Part model, mm, in its own coordinate system. A direction names the side the tool comes from. Round coordinates to 2 decimals unless told otherwise and drop trailing zeros. Loops run counter-clockwise (first coordinate to the right, second up) from the corner with the lowest first, then second, coordinate; pieces in that order, holes last. Notation, with made-up numbers: (48.5, 15) -> (94.5, 15) arc R25 cw to (94.5, 27) -> close; hole circle Ø8 at (58, -28.75). An arc over 180 degrees is marked (long way). Use a Markdown table: item, result. Add a question column.
Item 1: Probe line 1 (Y direction, x = 104.5, z = 25); line 2 (Y direction, x = 107.5, z = 35); line 3 (X direction, y = 83.5, z = 4.5). List the from-to ranges inside material, lowest first. Write a range as [from, to].
Item 2: Cut at C-C, the plane z = 13. List the corners of the cut face in (x, y), plus the area to 3 significant figures.
Item 3: Flat gauge pins, fed straight in: pin 1 (6.5 mm diameter, centred on y = 85, z = 25, fed in from +X); pin 2 (10.5 mm diameter, centred on y = 85, z = -25, fed in from -X); pin 3 (1.5 mm diameter, centred on x = 6, z = 24, fed in from +Y). Where does each tip first touch, or does it go through?
Item 4: Cut at A-A, the plane y = 95. List the corners of the cut face in (x, z).
Item 5: Cut at D-D, the plane y = 40. List the corners of the cut face in (x, z).
Item 6: Two-plate mould, pull along Z, no slides. Class faces 1 (the face through (28, 9, -40)), 2 (the face through (104.93, 32.11, -33.66)), 3 (the face through (4, 0, 1)), 4 (the face through (28, 9, 40)): pulls with the +Z half, pulls with the -Z half, needs draft (parallel to the pull), parting line crosses it, or undercut.
Item 7: Cut at B-B, the plane z = 35. List the corners of the cut face in (x, y), plus the area to 3 significant figures.
Item 8: Which spindle directions (+Z, -Z, +X, -X, +Y, -Y) get a long thin tool onto all of the face, cutting with end or side? Do faces 5 (the face through (104.93, 97.48, 34.67)), 6 (the face through (-1, 10, -1)). Say none if no direction does.
```python
from build123d import *

# Parameters (mm, degrees)
SKETCH2_W           = 200
SKETCH2_H           = 80
BOSS_EXTRUDE1_DEPTH = 10
SKETCH3_W           = 80
SKETCH3_H           = 100
BOSS_EXTRUDE2_DEPTH = 10
SKETCH6_R           = 4
CUT_EXTRUDE2_DEPTH  = 10
SKETCH8_R           = 2.5
CUT_EXTRUDE3_DEPTH  = 100


with BuildPart() as part:
    # Sketch2 → Boss-Extrude1 (new body)
    with BuildSketch(Plane(origin=(0, 0, 0), x_dir=(1, 0, 0), z_dir=(0, 1, 0))):
        Rectangle(SKETCH2_W, SKETCH2_H)
    extrude(amount=BOSS_EXTRUDE1_DEPTH)

    # Sketch3 → Boss-Extrude2 (add)
    with BuildSketch(Plane(origin=(100, 0, 0), x_dir=(0, 0, -1), z_dir=(1, 0, 0))):
        with Locations((0, 50)):
            Rectangle(SKETCH3_W, SKETCH3_H)
    extrude(amount=BOSS_EXTRUDE2_DEPTH)

    # Sketch6 → Cut-Extrude2 (cut)
    with BuildSketch(Plane.ZY.offset(-100)):
        with Locations((-25, 85)):
            Circle(SKETCH6_R)
        with Locations((25, 85)):
            Circle(SKETCH6_R)
        with Locations((-25, 40)):
            Circle(SKETCH6_R)
        with Locations((25, 40)):
            Circle(SKETCH6_R)
    extrude(amount=-CUT_EXTRUDE2_DEPTH, mode=Mode.SUBTRACT)

    # Sketch8 → Cut-Extrude3 (cut)
    with BuildSketch(Plane.ZY.offset(-100)):
        with Locations((-35, 95)):
            Circle(SKETCH8_R)
        with Locations((35, 95)):
            Circle(SKETCH8_R)
        with Locations((-35, 30)):
            Circle(SKETCH8_R)
        with Locations((35, 30)):
            Circle(SKETCH8_R)
    extrude(amount=-CUT_EXTRUDE3_DEPTH, mode=Mode.SUBTRACT)


solid = part.part
```
A:
| question | item | result |
|---|---|---|
| 1 | line 1 | y = [0, 36], [44, 81], [89, 100] |
| 1 | line 2 | y = [0, 27.5], [32.5, 92.5], [97.5, 100] |
| 1 | line 3 | x = [100, 110] |
| 2 | outline | (-100, 0) -> (110, 0) -> (110, 100) -> (100, 100) -> (100, 10) -> (-100, 10) -> close |
| 2 | area | 3,000 mm^2 |
| 3 | pin 1 | passes through |
| 3 | pin 2 | stops at x = 100 |
| 3 | pin 3 | stops at y = 10 |
| 4 | outline | (100, -40) -> (110, -40) -> (110, -37.5) -> (100, -37.5) -> close; (100, -32.5) -> (110, -32.5) -> (110, 32.5) -> (100, 32.5) -> close; (100, 37.5) -> (110, 37.5) -> (110, 40) -> (100, 40) -> close |
| 5 | outline | (100, -40) -> (110, -40) -> (110, -29) -> (100, -29) -> close; (100, -21) -> (110, -21) -> (110, 21) -> (100, 21) -> close; (100, 29) -> (110, 29) -> (110, 40) -> (100, 40) -> close |
| 6 | face 1 | pulls with the -Z half |
| 6 | face 2 | undercut |
| 6 | face 3 | needs draft |
| 6 | face 4 | pulls with the +Z half |
| 7 | outline | (-100, 0) -> (110, 0) -> (110, 27.5) -> (100, 27.5) -> (100, 10) -> (-100, 10) -> close; (100, 32.5) -> (110, 32.5) -> (110, 92.5) -> (100, 92.5) -> close; (100, 97.5) -> (110, 97.5) -> (110, 100) -> (100, 100) -> close |
| 7 | area | 2,900 mm^2 |
| 8 | face 5 | +X, -X |
| 8 | face 6 | +Z, -Z, -X, +Y |
